Here's the drawing with two shaded views (mm, measured from the low corner). I have some questions. A direction names the side the tool comes from. Coordinates: 2 decimals unless noted, no trailing zeros. Write each loop counter-clockwise with the first axis right and the second up, starting at its lowest first coordinate (ties: lowest second). Pieces come first, ordered by that corner, then holes. Notation, with made-up numbers: (5, 1) -> (45, 1) arc R27 cw to (45, 24) -> close; hole circle Ø3 at (28.5, 11). An arc over 180 degrees is marked (long way). Use one line per item in the form item = value.
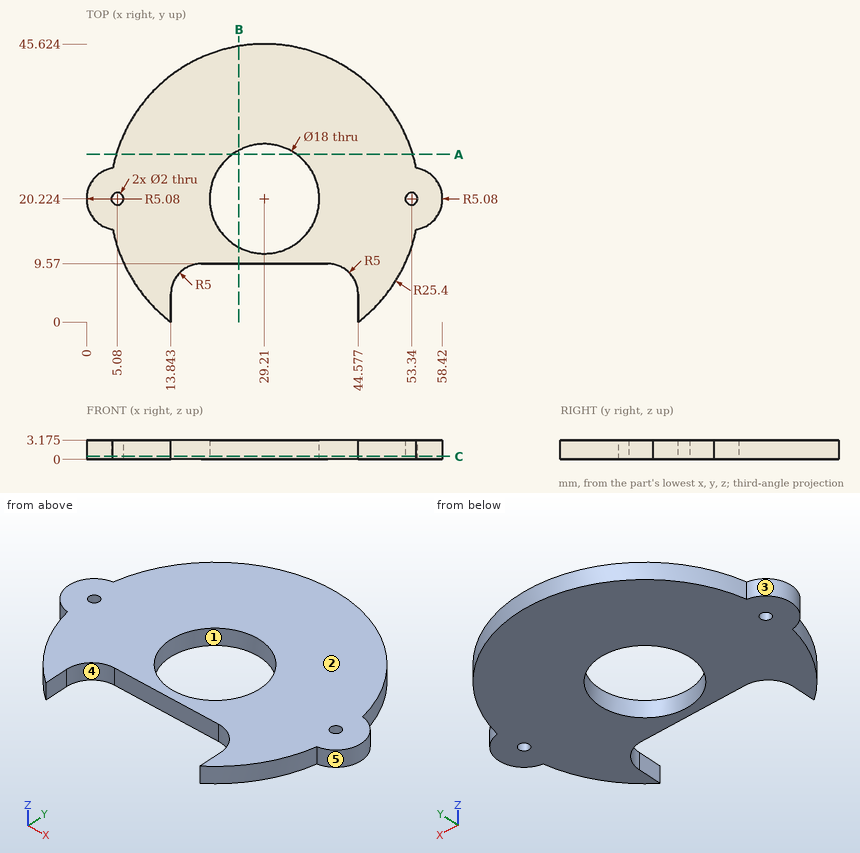
Q1. Will these pins go through, and if not, where does the flat tip stop? pin 1 (1.6 mm diameter, centred on y = 3.5, z = 1.5, fed in from -X); pin 2 (1.5 mm diameter, centred on x = 38.5, z = 1, fed in from +Y) (1 decimal); pin 3 (1.6 mm diameter, centred on x = 5.08, y = 20.22, fed in from -Z); pin 4 (1.5 mm diameter, centred on y = 23.5, z = 1.5, fed in from -X).
Return value:
pin_1 = 9.42
pin_2 = 44.1
pin_3 = through
pin_4 = 0.67
Q2. Suppose I cut it at C-C (z = 0.5). Write out the boundary of the cut face in (x, y) (1 decimal).
Return value:
outline = (4.3, 15.2) arc R25.4 ccw to (13.8, 0) -> (13.8, 4.6) arc R5 cw to (18.8, 9.6) -> (39.6, 9.6) arc R5 cw to (44.6, 4.6) -> (44.6, 0) arc R25.4 ccw to (54.1, 15.2) arc R5.1 ccw to (54.1, 25.2) arc R25.4 ccw to (4.3, 25.2) arc R5.1 ccw to start; hole circle Ø2 at (5.1, 20.2); hole circle Ø18 at (29.2, 20.2); hole circle Ø2 at (53.3, 20.2)
Q3. Thinking about a two-plate mould opening in X: for the marked faces 1, 2 and 3, which applies, released by +X, released by -X, zero draft, split by the parting line, or undercut?
Return value:
face_1 = undercut
face_2 = zero draft
face_3 = released by -X
Q4. Suppose I cut it at B-B (x = 25). Write out the boundary of the cut face in (y, z) (1 decimal).
Return value:
outline = (9.6, 0) -> (12.3, 0) -> (12.3, 3.2) -> (9.6, 3.2) -> close; (28.2, 0) -> (45.3, 0) -> (45.3, 3.2) -> (28.2, 3.2) -> close
Q5. For the marked faces 4 and 5, which set-ups out of +Z, -Z, +X, -X, +Y, -Y let a thin tool reach every point of the face, with its end or its side?
Return value:
face_4 = +Z, -Z, -Y
face_5 = +Z, -Z, +X
Q6. If I drill on line 1 (X direction, y = 26, z = 1.35) (1 decimal); line 2 (X direction, y = 18, z = 1); line 3 (Y direction, x = 23, z = 0.4) (1 decimal), over which ranges is the centre line in solid material (lowest first)? Write a range as from..to.
Return value:
line_1 = 4.5..22.3, 36.1..53.9
line_2 = 0.51..20.49, 37.93..57.91
line_3 = 9.6..13.7, 26.7..44.9
Q7. Suppose I cut it at A-A (y = 27.5). Write out the boundary of the cut face in (x, z) (1 decimal), then the cut area to 3 significant figures.
Return value:
outline = (4.9, 0) -> (23.9, 0) -> (23.9, 3.2) -> (4.9, 3.2) -> close; (34.5, 0) -> (53.5, 0) -> (53.5, 3.2) -> (34.5, 3.2) -> close
area = 121 mm2
